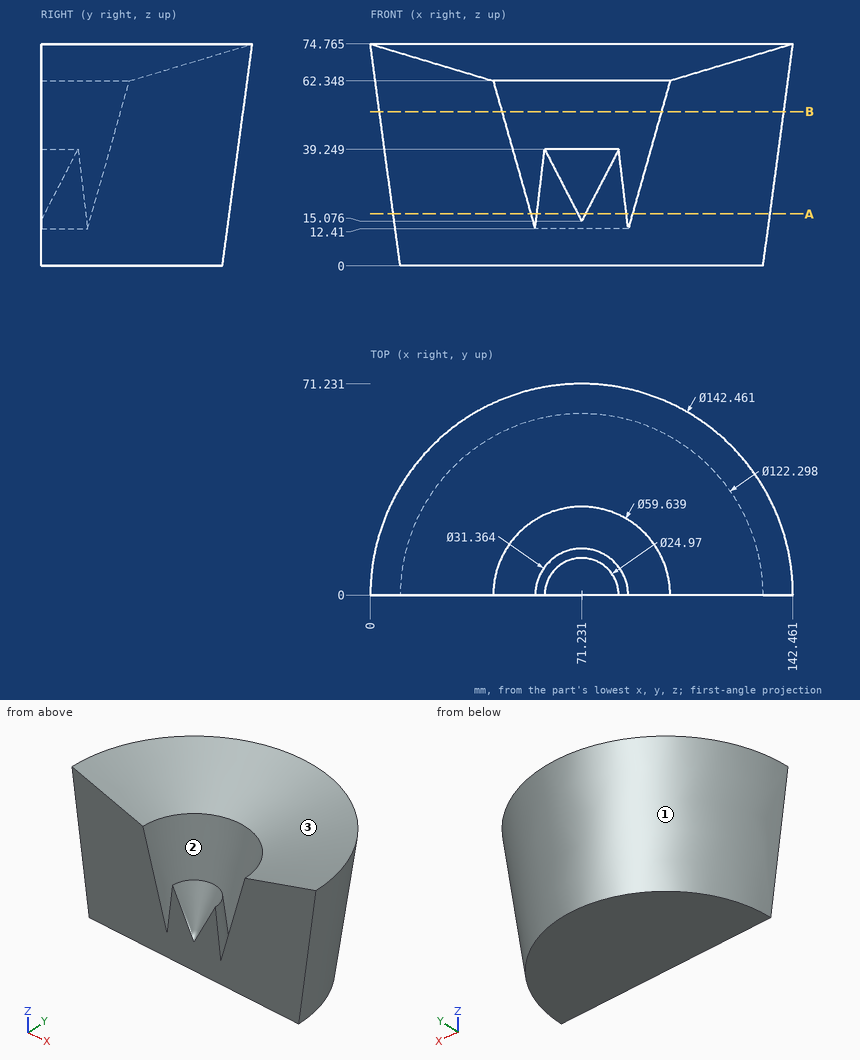
For this review, use the dimensioned drawing (mm, ordinates from the lowest corner) and the shaded views. Round coordinates to 2 decimals unless told otherwise and drop trailing zeros. Order: outer loops, then holes, each group sorted by start corner. A loop starts at its lowest first (then second) coordinate and runs counter-clockwise, first axis right, second up. Notation, with made-up numbers: M 35,18.5 L 39,18.5 A19 ccw 39,48.5 Z; hole C 49,3 d2. An arc over 180 degrees is marked long. Use a Markdown table: item, result.
1) Consider section B-B (z = 52). Write out the cut boundary in (x, y), then the cut area to 3 significant figures.
Report:
| item | result |
|---|---|
| outline | M 3.07,0 L 44.34,0 A26.89 cw 98.12,0 L 139.39,0 A68.16 ccw Z |
| area | 6,160 mm^2 |
2) Wall thickness on line 1 along X through (y, z) = (8, 15) (1 decimal); line 2 along X through (y, z) = (8, 26) (1 decimal); line 3 along X through (y, z) = (37.5, 35.5) (1 decimal): over which ranges is each line inside the solid? List them lowest first. Write a range as [from, to].
Report:
| item | result |
|---|---|
| line 1 | [8.6, 56.9], [58.1, 84.4], [85.6, 133.9] |
| line 2 | [7.1, 53.4], [59.7, 82.8], [89, 135.4] |
| line 3 | [17, 125.5] |
3) Insertion check: pin 1 (8 mm diameter, centred on x = 122, z = 8.5, fed in from +Y); pin 2 (5 mm diameter, centred on y = 22, z = 27, fed in from +X); pin 3 (1 mm diameter, centred on x = 33.5, y = 44, fed in from +Z). Each pin has a flat end and moves straight along its axis. Give the tip position at first contact, or say it passes through.
Report:
| item | result |
|---|---|
| pin 1 | y = 41.22 |
| pin 2 | x = 133.09 |
| pin 3 | z = 70.94 |
4) Draft analysis for pull direction Y (two halves, no side actions). For the marked faces 1, 2 and 3, state which applies: released by +Y, released by -Y, zero draft, split by the parting line, or undercut.
Report:
| item | result |
|---|---|
| face 1 | released by +Y |
| face 2 | undercut |
| face 3 | released by -Y |
5) Consider section A-A (z = 17.5). Write out the cut boundary in (x, y) (1 decimal), then the cut area to 3 significant figures.
Report:
| item | result |
|---|---|
| outline | M 7.7,0 L 54.1,0 A17.1 cw 88.4,0 L 134.7,0 A63.5 ccw Z; M 56.2,0 L 70,0 A1.3 cw 72.5,0 L 86.3,0 A15.1 ccw Z |
| area | 6,230 mm^2 |
